CAD build for the part. Positions are in the model's coordinates, mm. Coordinates: 2 decimals unless noted, no trailing zeros. Write each loop counter-clockwise with the first axis right and the second up, starting at its lowest first coordinate (ties: lowest second). Pieces come first, ordered by that corner, then holes. Notation, with made-up numbers: M 18,0 L 42,0 A20 ccw 42,21 Z; hole C 73.5,7.25 d1. An arc over 180 degrees is marked long. Put each result on its own line as item: value. Start each with the question number.
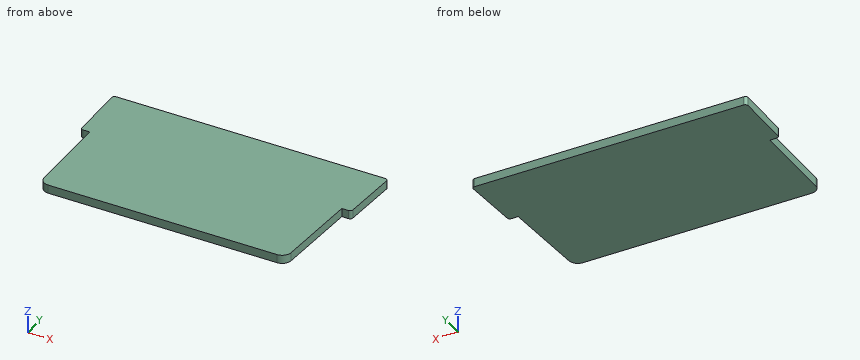
```python
from build123d import *

# Parameters (mm, degrees)
F1_DEPTH = 1.524
F2_R     = 0.508
F3_R     = 1.651


with BuildPart() as f1:
    # F0 (on Top) → F1 (new body)
    with BuildSketch(Plane.XY):
        Polygon((-22.987, 17.018), (-22.479, 0), (22.479, 0), (22.987, 17.018), (24.7015, 17.018), (25.0825, 28.194), (-25.0825, 28.194), (-24.7015, 17.018), align=None)
    extrude(amount=F1_DEPTH)

    # F2
    f2_edges = [f1.edges().sort_by_distance(p)[0] for p in [
        (25.0825, 28.194, 0.762),
        (24.7015, 17.018, 0.762),
        (-25.0825, 28.194, 0.762),
        (-24.7015, 17.018, 0.762),
    ]]
    fillet(f2_edges, radius=F2_R)

    # F3
    f3_edges = [f1.edges().sort_by_distance(p)[0] for p in [
        (-22.479, 0, 0.762),
        (22.479, 0, 0.762),
    ]]
    fillet(f3_edges, radius=F3_R)


solid = f1.part
```
(1) Slice it at A-A, the plane z = 0.8. Write the cut outline in (x, y), then the cut area to 3 significant figures.
(2) Slice it at B-B, the plane y = 15.25. Write the cut outline in (x, z), then the cut area to 3 significant figures.
(3) Slice it at C-C, the plane y = 9. Write the cut outline in (x, z).
(4) Drill centre lines: line 1 (X direction, y = 22, z = 1.25); line 2 (X direction, y = 5, z = 1.05). Where is each one in solid material? Low to high. Write a range as [from, to].
Result set:
1. outline: M -25.06,27.67 L -24.72,17.51 A0.51 ccw -24.21,17.02 L -22.99,17.02 L -22.53,1.6 A1.65 ccw -20.88,0 L 20.88,0 A1.65 ccw 22.53,1.6 L 22.99,17.02 L 24.21,17.02 A0.51 ccw 24.72,17.51 L 25.06,27.67 A0.51 ccw 24.56,28.19 L -24.56,28.19 A0.51 ccw Z
1. area: 1,330 mm^2
2. outline: M -22.93,0 L 22.93,0 L 22.93,1.52 L -22.93,1.52 Z
2. area: 69.9 mm^2
3. outline: M -22.75,0 L 22.75,0 L 22.75,1.52 L -22.75,1.52 Z
4. line 1: x = [-24.87, 24.87]
4. line 2: x = [-22.63, 22.63]
